Input: part model. Units: mm. Frame: model coordinates. Face numbers are marked on the shaded views. A direction names the side the tool comes from. Coordinates: 2 decimals unless noted, no trailing zeros. Order: outer loops, then holes, each group sorted by start corner. A loop starts at its lowest first (then second) coordinate and runs counter-clockwise, first axis right, second up. Notation, with made-up numbers: (44, 79.5) -> (49, 79.5) arc R17 cw to (49, 111.5) -> close; hole circle Ø2 at (-10, -36.75). An arc over 180 degrees is marked (long way). Write each question's results on one line, items separated by ' | '.
```python
from build123d import *

# Parameters (mm, degrees)
SKETCH1_W            = 160
SKETCH1_H            = 221
BOSS_EXTRUDE2_DEPTH  = 74
CUT_EXTRUDE2_DEPTH   = 164
SKETCH8_W            = 152
SKETCH8_H            = 156
CUT_EXTRUDE3_DEPTH   = 72
SKETCH10_W           = 152
SKETCH10_H           = 72
CUT_EXTRUDE4_DEPTH   = 57
SKETCH12_W           = 4.5
SKETCH12_H           = 4.5
BOSS_EXTRUDE3_DEPTH  = 72
SKETCH13_W           = 4.5
SKETCH13_H           = 4.5
BOSS_EXTRUDE4_DEPTH  = 80
CUT_EXTRUDE5_DEPTH   = 80
CUT_EXTRUDE6_DEPTH   = 80
SKETCH18_W           = 90
SKETCH18_H           = 58
BOSS_EXTRUDE6_DEPTH  = 72
SKETCH21_W           = 86
SKETCH21_H           = 54
CUT_EXTRUDE7_DEPTH   = 72
SKETCH22_W           = 4
SKETCH22_H           = 4
BOSS_EXTRUDE7_DEPTH  = 72
SKETCH24_R           = 2.25
CUT_EXTRUDE8_DEPTH   = 5.9
SKETCH25_W           = 62.3
SKETCH25_H           = 20.1
BOSS_EXTRUDE8_DEPTH  = 16.5
FILLET1_R            = 3
FILLET2_R            = 3
FILLET3_R            = 2
FILLET4_R            = 2
SKETCH28_W           = 19.81
SKETCH28_H           = 10.54
BOSS_EXTRUDE10_DEPTH = 6.35
SKETCH29_W           = 2.5
SKETCH29_H           = 10.54
SKETCH29_W_2         = 2.4979753
BOSS_EXTRUDE11_DEPTH = 22.35
SKETCH33_R           = 3.45
CUT_EXTRUDE11_DEPTH  = 22.35
SKETCH34_R           = 1.55
SKETCH34_W           = 27.4
SKETCH34_H           = 19.4
CUT_EXTRUDE12_DEPTH  = 10
SKETCH44_R           = 1.5
CUT_EXTRUDE13_DEPTH  = 52
SKETCH47_R           = 1.5
CUT_EXTRUDE15_DEPTH  = 52
SKETCH48_R           = 1.5
CUT_EXTRUDE16_DEPTH  = 52
CUT_EXTRUDE19_START  = 15
SKETCH52_R           = 1.5
CUT_EXTRUDE19_DEPTH  = 69
SKETCH54_R           = 1.5
CUT_EXTRUDE20_DEPTH  = 52
SKETCH65_R           = 3.15
BOSS_EXTRUDE16_DEPTH = 10
SKETCH66_R           = 1.5
CUT_EXTRUDE24_DEPTH  = 15
SKETCH67_R           = 1.5
CUT_EXTRUDE25_DEPTH  = 15
SKETCH68_W           = 25
SKETCH68_H           = 37
CUT_EXTRUDE26_DEPTH  = 15
SKETCH69_W           = 2
SKETCH69_H           = 37
BOSS_EXTRUDE18_DEPTH = 4


with BuildPart() as part:
    # Sketch1 → Boss-Extrude2 (new body)
    with BuildSketch(Plane(origin=(0, 0, 0), x_dir=(1, 0, 0), z_dir=(0, 1, 0))):
        with Locations((0, -30.5)):
            Rectangle(SKETCH1_W, SKETCH1_H)
    extrude(amount=BOSS_EXTRUDE2_DEPTH)

    # Sketch7 → Cut-Extrude2 (cut)
    with BuildSketch(Plane(origin=(80, 0, 0), x_dir=(0, 0, -1), z_dir=(1, 0, 0))):
        Polygon((-141, 74), (-80, 74), (-141, 39), align=None)
    extrude(amount=-CUT_EXTRUDE2_DEPTH, mode=Mode.SUBTRACT)

    # Sketch8 → Cut-Extrude3 (cut)
    with BuildSketch(Plane(origin=(0, 74, 0), x_dir=(1, 0, 0), z_dir=(0, 1, 0))):
        with Locations((0, -2)):
            Rectangle(SKETCH8_W, SKETCH8_H)
    extrude(amount=-CUT_EXTRUDE3_DEPTH, mode=Mode.SUBTRACT)

    # Sketch10 → Cut-Extrude4 (cut)
    with BuildSketch(Plane(origin=(0, 0, 80), x_dir=(-1, 0, 0), z_dir=(0, 0, -1))):
        with Locations((0, 38)):
            Rectangle(SKETCH10_W, SKETCH10_H)
    extrude(amount=-CUT_EXTRUDE4_DEPTH, mode=Mode.SUBTRACT)

    # Sketch12 → Boss-Extrude3 (add)
    with BuildSketch(Plane(origin=(0, 2, 0), x_dir=(1, 0, 0), z_dir=(0, 1, 0))):
        with Locations((-73.75, 73.75)):
            Rectangle(SKETCH12_W, SKETCH12_H)
        with Locations((73.75, 73.75)):
            Rectangle(SKETCH12_W, SKETCH12_H)
        with Locations((-73.75, -77.75)):
            Rectangle(SKETCH12_W, SKETCH12_H)
        with Locations((73.75, -77.75)):
            Rectangle(SKETCH12_W, SKETCH12_H)
    extrude(amount=BOSS_EXTRUDE3_DEPTH)

    # Sketch13 → Boss-Extrude4 (add)
    with BuildSketch(Plane(origin=(0, 2, 0), x_dir=(1, 0, 0), z_dir=(0, 1, 0))):
        with Locations((-73.75, -82.25)):
            Rectangle(SKETCH13_W, SKETCH13_H)
        with Locations((-73.75, -134.75)):
            Rectangle(SKETCH13_W, SKETCH13_H)
        with Locations((73.75, -82.25)):
            Rectangle(SKETCH13_W, SKETCH13_H)
        with Locations((73.75, -134.75)):
            Rectangle(SKETCH13_W, SKETCH13_H)
    extrude(amount=BOSS_EXTRUDE4_DEPTH)

    # Sketch14 → Cut-Extrude5 (cut)
    with BuildSketch(Plane.ZY.offset(76)):
        Polygon((80, 82), (84.5, 82), (84.5, 71.418032787), (80, 74), align=None)
        Polygon((137, 41.295081967), (132.5, 43.87704918), (132.5, 82), (137, 82), align=None)
    extrude(amount=-CUT_EXTRUDE5_DEPTH, mode=Mode.SUBTRACT)

    # Sketch15 → Cut-Extrude6 (cut)
    with BuildSketch(Plane(origin=(76, 0, 0), x_dir=(0, 0, -1), z_dir=(1, 0, 0))):
        Polygon((-137, 41.295081967), (-132.5, 43.87704918), (-132.5, 82), (-137, 82), align=None)
        Polygon((-84.5, 71.418032787), (-80, 74), (-80, 82), (-84.5, 82), align=None)
    extrude(amount=-CUT_EXTRUDE6_DEPTH, mode=Mode.SUBTRACT)

    # Sketch18 → Boss-Extrude6 (add)
    with BuildSketch(Plane(origin=(0, 2, 0), x_dir=(1, 0, 0), z_dir=(0, 1, 0))):
        with Locations((31, 47)):
            Rectangle(SKETCH18_W, SKETCH18_H)
    extrude(amount=BOSS_EXTRUDE6_DEPTH)

    # Sketch21 → Cut-Extrude7 (cut)
    with BuildSketch(Plane(origin=(0, 74, 0), x_dir=(1, 0, 0), z_dir=(0, 1, 0))):
        with Locations((33, 49)):
            Rectangle(SKETCH21_W, SKETCH21_H)
    extrude(amount=-CUT_EXTRUDE7_DEPTH, mode=Mode.SUBTRACT)

    # Sketch22 → Boss-Extrude7 (add)
    with BuildSketch(Plane(origin=(0, 2, 0), x_dir=(1, 0, 0), z_dir=(0, 1, 0))):
        with Locations((74, 74)):
            Rectangle(SKETCH22_W, SKETCH22_H)
    extrude(amount=BOSS_EXTRUDE7_DEPTH)

    # Sketch24 → Cut-Extrude8 (cut)
    with BuildSketch(Plane.ZY.offset(14)):
        with Locations((-68.205440171, 13.198688186)):
            Circle(SKETCH24_R)
        with Locations((-68.205440171, 20.198688186)):
            Circle(SKETCH24_R)
    extrude(amount=-CUT_EXTRUDE8_DEPTH, mode=Mode.SUBTRACT)

    # Sketch25 → Boss-Extrude8 (add)
    with BuildSketch(Plane(origin=(0, 2, 0), x_dir=(1, 0, 0), z_dir=(0, 1, 0))):
        with Locations((34.15, 40.95)):
            Rectangle(SKETCH25_W, SKETCH25_H)
    extrude(amount=BOSS_EXTRUDE8_DEPTH)

    # Fillet1
    fillet1_edges = [part.edges().sort_by_distance(p)[0] for p in [
        (80, 37, -80),
    ]]
    fillet(fillet1_edges, radius=FILLET1_R)

    # Fillet2
    fillet2_edges = [part.edges().sort_by_distance(p)[0] for p in [
        (-80, 37, -80),
    ]]
    fillet(fillet2_edges, radius=FILLET2_R)

    # Fillet3
    fillet3_edges = [part.edges().sort_by_distance(p)[0] for p in [
        (80, 19.5, 141),
    ]]
    fillet(fillet3_edges, radius=FILLET3_R)

    # Fillet4
    fillet4_edges = [part.edges().sort_by_distance(p)[0] for p in [
        (-80, 19.5, 141),
    ]]
    fillet(fillet4_edges, radius=FILLET4_R)

    # Sketch28 → Boss-Extrude10 (add)
    with BuildSketch(Plane(origin=(0, 2, 0), x_dir=(1, 0, 0), z_dir=(0, 1, 0))):
        with Locations((-51.085, -131.73)):
            Rectangle(SKETCH28_W, SKETCH28_H)
        with Locations((-26.085, -131.73)):
            Rectangle(SKETCH28_W, SKETCH28_H)
    extrude(amount=BOSS_EXTRUDE10_DEPTH)

    # Sketch29 → Boss-Extrude11 (add)
    with BuildSketch(Plane(origin=(0, 2, 0), x_dir=(1, 0, 0), z_dir=(0, 1, 0))):
        with Locations((-61.14, -131.73)):
            Rectangle(SKETCH29_W, SKETCH29_H)
        with Locations((-41.03, -131.73)):
            Rectangle(SKETCH29_W, SKETCH29_H)
        with Locations((-36.14, -131.73)):
            Rectangle(SKETCH29_W, SKETCH29_H)
        with Locations((-16.03101235, -131.73)):
            Rectangle(SKETCH29_W_2, SKETCH29_H)
    extrude(amount=BOSS_EXTRUDE11_DEPTH)

    # Sketch33 → Cut-Extrude11 (cut)
    with BuildSketch(Plane(origin=(0, 0, 137), x_dir=(-1, 0, 0), z_dir=(0, 0, -1))):
        with Locations((51.187629476, 16.178708102)):
            Circle(SKETCH33_R)
        with Locations((26.187629476, 16.178708102)):
            Circle(SKETCH33_R)
    extrude(amount=-CUT_EXTRUDE11_DEPTH, mode=Mode.SUBTRACT)

    # Sketch34 → Cut-Extrude12 (cut)
    with BuildSketch(Plane.XY.offset(-76)):
        with Locations((64.8, 15.464095432)):
            Circle(SKETCH34_R)
        with Locations((26.8, 15.4)):
            Circle(SKETCH34_R)
        with Locations((45.8, 15.2)):
            Rectangle(SKETCH34_W, SKETCH34_H)
    extrude(amount=-CUT_EXTRUDE12_DEPTH, mode=Mode.SUBTRACT)

    # Sketch44 → Cut-Extrude13 (cut)
    with BuildSketch(Plane(origin=(0, 74, 0), x_dir=(1, 0, 0), z_dir=(0, 1, 0))):
        with Locations(Location((-73.75, 73.75, 0), (0, 0, 270))):
            Circle(SKETCH44_R)
    extrude(amount=-CUT_EXTRUDE13_DEPTH, mode=Mode.SUBTRACT)

    # Sketch47 → Cut-Extrude15 (cut)
    with BuildSketch(Plane(origin=(0, 74, 0), x_dir=(1, 0, 0), z_dir=(0, 1, 0))):
        with Locations(Location((74.25, 74.25, 0), (0, 0, 270))):
            Circle(SKETCH47_R)
    extrude(amount=-CUT_EXTRUDE15_DEPTH, mode=Mode.SUBTRACT)

    # Sketch48 → Cut-Extrude16 (cut)
    with BuildSketch(Plane(origin=(0, 74, 0), x_dir=(1, 0, 0), z_dir=(0, 1, 0))):
        with Locations(Location((73.75, -77.75, 0), (0, 0, 270))):
            Circle(SKETCH48_R)
    extrude(amount=-CUT_EXTRUDE16_DEPTH, mode=Mode.SUBTRACT)

    # Sketch52 → Cut-Extrude19 (cut)
    with BuildSketch(Plane(origin=(0, 2, 0), x_dir=(1, 0, 0), z_dir=(0, 1, 0)).offset(CUT_EXTRUDE19_START)):
        with Locations(Location((73.75, -82.25, 0), (0, 0, 270))):
            Circle(SKETCH52_R)
        with Locations(Location((-73.75, -82.25, 0), (0, 0, 270))):
            Circle(SKETCH52_R)
        with Locations(Location((-73.75, -134.75, 0), (0, 0, 270))):
            Circle(SKETCH52_R)
        with Locations(Location((73.75, -134.75, 0), (0, 0, 270))):
            Circle(SKETCH52_R)
    extrude(amount=CUT_EXTRUDE19_DEPTH, mode=Mode.SUBTRACT)

    # Sketch54 → Cut-Extrude20 (cut)
    with BuildSketch(Plane(origin=(0, 74, 0), x_dir=(1, 0, 0), z_dir=(0, 1, 0))):
        with Locations(Location((-73.75, -77.75, 0), (0, 0, 270))):
            Circle(SKETCH54_R)
    extrude(amount=-CUT_EXTRUDE20_DEPTH, mode=Mode.SUBTRACT)

    # Sketch65 → Boss-Extrude16 (add)
    with BuildSketch(Plane.XY.offset(-76)):
        with Locations(Location((26.859149397, 15.23123202, 0), (0, 0, 180))):
            Circle(SKETCH65_R)
        with Locations(Location((64.799149397, 15.23123202, 0), (0, 0, 180))):
            Circle(SKETCH65_R)
    extrude(amount=BOSS_EXTRUDE16_DEPTH)

    # Sketch66 → Cut-Extrude24 (cut)
    with BuildSketch(Plane.XY.offset(-76)):
        with Locations(Location((26.840517017, 15.277397511, 0), (0, 0, 218.813706581))):
            Circle(SKETCH66_R)
    extrude(amount=CUT_EXTRUDE24_DEPTH, mode=Mode.SUBTRACT)

    # Sketch67 → Cut-Extrude25 (cut)
    with BuildSketch(Plane.XY.offset(-76)):
        with Locations(Location((64.952271836, 15.4, 0), (0, 0, 261.804750978))):
            Circle(SKETCH67_R)
    extrude(amount=CUT_EXTRUDE25_DEPTH, mode=Mode.SUBTRACT)

    # Sketch68 → Cut-Extrude26 (cut)
    with BuildSketch(Plane(origin=(80, 0, 0), x_dir=(0, 0, -1), z_dir=(1, 0, 0))):
        with Locations((-10.266957333, 36.517419115)):
            Rectangle(SKETCH68_W, SKETCH68_H)
        with Locations((49.733042667, 36.517419115)):
            Rectangle(SKETCH68_W, SKETCH68_H)
    extrude(amount=-CUT_EXTRUDE26_DEPTH, mode=Mode.SUBTRACT)

    # Sketch69 → Boss-Extrude18 (add)
    with BuildSketch(Plane(origin=(80, 0, 0), x_dir=(0, 0, -1), z_dir=(1, 0, 0))):
        with Locations((40.733042667, 36.517419115)):
            Rectangle(SKETCH69_W, SKETCH69_H)
        with Locations((45.233042667, 36.517419115)):
            Rectangle(SKETCH69_W, SKETCH69_H)
        with Locations((49.733042667, 36.517419115)):
            Rectangle(SKETCH69_W, SKETCH69_H)
        with Locations((54.233042667, 36.517419115)):
            Rectangle(SKETCH69_W, SKETCH69_H)
        with Locations((58.733042667, 36.517419115)):
            Rectangle(SKETCH69_W, SKETCH69_H)
        with Locations((-19.266957333, 36.517419115)):
            Rectangle(SKETCH69_W, SKETCH69_H)
        with Locations((-14.766957333, 36.517419115)):
            Rectangle(SKETCH69_W, SKETCH69_H)
        with Locations((-10.266957333, 36.517419115)):
            Rectangle(SKETCH69_W, SKETCH69_H)
        with Locations((-5.766957333, 36.517419115)):
            Rectangle(SKETCH69_W, SKETCH69_H)
        with Locations((-1.266957333, 36.517419115)):
            Rectangle(SKETCH69_W, SKETCH69_H)
    extrude(amount=-BOSS_EXTRUDE18_DEPTH)


solid = part.part
```
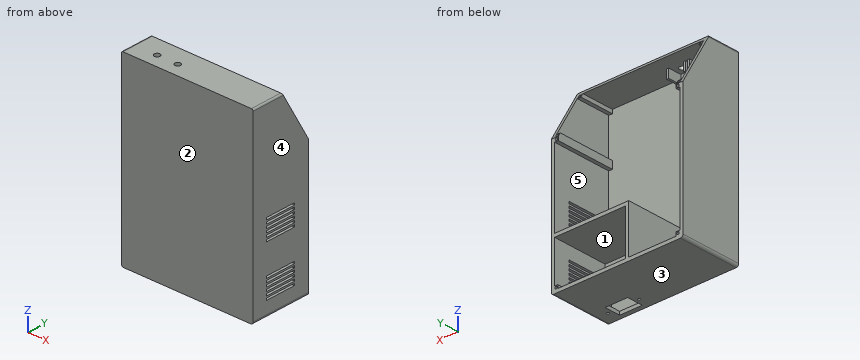
(1) Cut plane C-C, the plane y = 28. Count the separate pieces of the cut face and the enclosed holes in it, plus the area to 3 significant figures.
Return value:
separate pieces: 11 | enclosed holes: 8 | area: 3,540 mm2
(2) Pin query (flat end, axial travel): P1, Ø1.3, axis at x = 65, y = 15, coming from the -Z side; P2, Ø4.5, axis at x = 78.5, y = 38.5, coming from the +Z side; P3, Ø1, axis at x = 59, z = 29.5, coming from the +Y side; P4, Ø2, axis at x = 13.5, y = 50.5, coming from the +Z side. Return the tip coordinate at first contact, or that it passes through.
Return value:
P1: z = -51 | P2: z = 141 | P3: y = 2 | P4: z = -18
(3) Mould query, pull axis X, two halves, no side actions, for the marked faces 3, 4 and 5. Classes: +X half, -X half, draft (parallel to the pull), parting line (faces both ways), or undercut.
Return value:
face 3: draft | face 4: +X half | face 5: undercut
(4) Reachability of the marked faces 1 and 2 from +Z, -Z, +X, -X, +Y, -Y: full face, straight path, thin tool, end or side. Return the list, or none.
Return value:
face 1: +Y | face 2: +Z, -Z, +X, -X, -Y
(5) Line query: line 1 along X through (y, z) = (59.5, 82.25); line 2 along Z through (x, y) = (12, 4.5); line 3 along X through (y, z) = (13.5, -25). Output: solid intervals per line, ascending. Write a range as from..to.
Return value:
line 1: -80..-75.25, -72.25..-71.5, 71.5..72.25, 75.25..80 | line 2: -80..-76, -51..-30.9, -22..-18, 137..141 | line 3: -80..-76, -14..-10, 76..80
(6) Cut plane A-A, the plane x = 43.5. Return loops of the section in (y, z).
Return value:
outline: (0, -80) -> (5.5, -80) -> (5.5, -76) -> (2, -76) -> (2, -51) -> (18.5, -51) -> (18.5, -30.9) -> (2, -30.9) -> (2, -22) -> (74, -22) -> (74, -18) -> (2, -18) -> (2, 137) -> (41.3, 137) -> (39, 141) -> (0, 141) -> close; (24.9, -80) -> (74, -80) -> (74, -76) -> (24.9, -76) -> close
(7) Cut plane B-B, the plane z = -33.5. Return loops of the section in (x, y), plus the area to 3 significant figures.
Return value:
outline: (-80, 0) -> (80, 0) -> (80, 74) -> (76, 74) -> (76, 2) -> (65.3, 2) -> (65.3, 18.5) -> (3, 18.5) -> (3, 2) -> (-10, 2) -> (-10, 74) -> (-14, 74) -> (-14, 2) -> (-76, 2) -> (-76, 74) -> (-80, 74) -> close | area: 2,210 mm2
(8) Cut plane D-D, the plane z = 67.5. Return loops of the section in (x, y), plus the area to 3 significant figures.
Return value:
outline: (-80, 0) -> (80, 0) -> (80, 74) -> (76, 74) -> (76, 2) -> (-76, 2) -> (-76, 74) -> (-80, 74) -> close | area: 896 mm2
